Part model, mm, in its own coordinate system. Face numbers are marked on the shaded views. Round coordinates to 2 decimals unless told otherwise and drop trailing zeros. Loops run counter-clockwise (first coordinate to the right, second up) from the corner with the lowest first, then second, coordinate; pieces in that order, holes last. Notation, with made-up numbers: (-38, 47) -> (-19, 47) arc R13 cw to (-19, 69) -> close; hole circle Ø2 at (-4, 10). An arc over 180 degrees is marked (long way). Answer as a JSON object with one key per item and string values. Group by question number.
from build123d import *

# Parameters (mm, degrees)
F0_R     = 3
F1_DEPTH = 0.8
F2_R     = 2.5
F3_DEPTH = 10
F4_R     = 1.25
F5_DEPTH = 25
F6_R     = 1.55
F6_R_2   = 1.25
F7_DEPTH = 1


with BuildPart() as f1:
    # F0 (on Front) → F1 (new body)
    with BuildSketch(Plane.XZ):
        Circle(F0_R)
    extrude(amount=F1_DEPTH)

    # F2 (on face) → F3 (join)
    with BuildSketch(Plane.XZ.offset(0.8)):
        Circle(F2_R)
    extrude(amount=F3_DEPTH)

    # F4 (on face) → F5 (cut)
    with BuildSketch(Plane.XZ.offset(10.8)):
        Circle(F4_R)
    extrude(amount=-F5_DEPTH, mode=Mode.SUBTRACT)

    # F6 (on face) → F7 (cut)
    with BuildSketch(Plane(origin=(0, 0, 0), x_dir=(-1, 0, 0), z_dir=(0, 1, 0))):
        Circle(F6_R)
        Circle(F6_R_2, mode=Mode.SUBTRACT)
        Circle(F6_R)
    extrude(amount=-F7_DEPTH, mode=Mode.SUBTRACT)


solid = f1.part
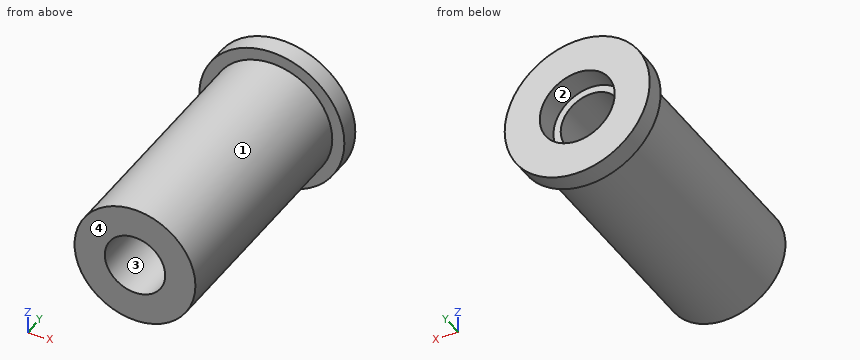
Item 1: Band-saw the part on A-A, the plane z = 0. List the corners of the cut face in (x, y), plus the area to 3 significant figures.
Item 2: Drill centre lines: line 1 (Z direction, x = 0, y = -8); line 2 (Z direction, x = 0, y = -0.55). Where is each one in solid material? Low to high.
Item 3: Band-saw the part on D-D, the plane y = -5.75. List the corners of the cut face in (x, z).
Item 4: Band-saw the part on C-C, the plane x = 1.7. List the corners of the cut face in (y, z).
Item 5: Two-plate mould, pull along X, no slides. Class the marked faces 1, 2, 3 and 4: pulls with the +X half, pulls with the -X half, needs draft (parallel to the pull), parting line crosses it, or undercut.
Item 6: Band-saw the part on B-B, the plane x = 0. List the corners of the cut face in (y, z).
Item 7: Drop flat-ended pins along their axis: pin 1 Ø3 at (x, z) = (0, 0) entering from +Y; pin 2 Ø1.5 at (y, z) = (-7.5, -1) entering from -X; pin 3 Ø1 at (y, z) = (-9.5, -1) entering from +X. Give the stop position or say it passes through.
Entries:
{
 "1": {"outline": "(-3, -0.8) -> (-2.5, -0.8) -> (-2.5, -10.8) -> (-1.25, -10.8) -> (-1.25, -1) -> (-1.55, -1) -> (-1.55, 0) -> (-3, 0) -> close; (1.25, -10.8) -> (2.5, -10.8) -> (2.5, -0.8) -> (3, -0.8) -> (3, 0) -> (1.55, 0) -> (1.55, -1) -> (1.25, -1) -> close", "area": "27.2 mm²"},
 "2": {"line 1": "-2.5 to -1.25, 1.25 to 2.5", "line 2": "-3 to -1.55, 1.55 to 3"},
 "3": {"outline": "circle Ø5 at (0, 0); hole circle Ø2.5 at (0, 0)"},
 "4": {"outline": "(-10.8, -1.83) -> (-0.8, -1.83) -> (-0.8, -2.47) -> (0, -2.47) -> (0, 2.47) -> (-0.8, 2.47) -> (-0.8, 1.83) -> (-10.8, 1.83) -> close"},
 "5": {"face 1": "parting line crosses it", "face 2": "undercut", "face 3": "undercut", "face 4": "needs draft"},
 "6": {"outline": "(-10.8, -2.5) -> (-0.8, -2.5) -> (-0.8, -3) -> (0, -3) -> (0, -1.55) -> (-1, -1.55) -> (-1, -1.25) -> (-10.8, -1.25) -> close; (-10.8, 1.25) -> (-1, 1.25) -> (-1, 1.55) -> (0, 1.55) -> (0, 3) -> (-0.8, 3) -> (-0.8, 2.5) -> (-10.8, 2.5) -> close"},
 "7": {"pin 1": "y = -1", "pin 2": "x = -2.49", "pin 3": "x = 2.45"}
}
